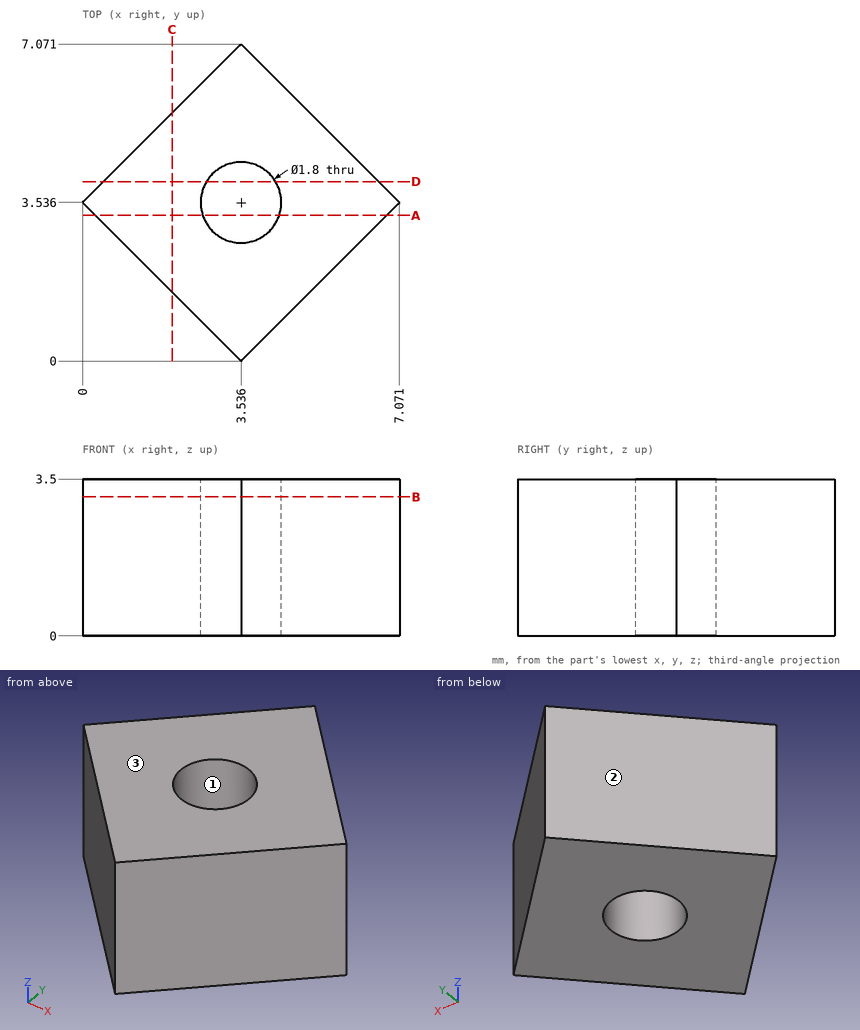
Here's the drawing with two shaded views (mm, measured from the low corner). I have some questions. Round coordinates to 2 decimals unless told otherwise and drop trailing zeros. Write each loop counter-clockwise with the first axis right and the second up, starting at its lowest first coordinate (ties: lowest second). Pieces come first, ordered by that corner, then holes. Notation, with made-up numbers: M 18,-10 L 22,-10 A29 cw 22,11 Z; hole C -12.5,-34.75 d2. An arc over 180 degrees is marked long. Use CSV: the item, a comma, the result in double quotes.
(1) I need wall thicknesses on line 1 along Y through (x, z) = (3.75, 3.3) (1 decimal); line 2 along Y through (x, z) = (3.25, 3.1) (1 decimal); line 3 along Y through (x, z) = (2.5, 0.85) (1 decimal). Which ranges of each line are inside material? Lowest first, please.
Check values:
line 1,"0.2 to 2.7, 4.4 to 6.9"
line 2,"0.3 to 2.7, 4.4 to 6.8"
line 3,"1 to 6"
(2) Imagine slicing it at B-B (z = 3.1). Write out the boundary of the cut face in (x, y) (1 decimal).
Check values:
outline,"M 0,3.5 L 3.5,0 L 7.1,3.5 L 3.5,7.1 Z; hole C 3.5,3.5 d1.8"
(3) Imagine slicing it at C-C (x = 2). Write out the boundary of the cut face in (y, z) (1 decimal).
Check values:
outline,"M 1.5,0 L 5.5,0 L 5.5,3.5 L 1.5,3.5 Z"
(4) I'm going to push flat-ended pins straight in: pin 1 (1.5 mm diameter, centred on x = 4, z = 1.5, fed in from +Y); pin 2 (1.6 mm diameter, centred on x = 3.54, y = 3.54, fed in from -Z); pin 3 (2 mm diameter, centred on y = 6, z = 3, fed in from +X) (1 decimal); pin 4 (2 mm diameter, centred on y = 5.5, z = 0.5, fed in from +X) (1 decimal). Where does each tip first touch, or does it pass through?
Check values:
pin 1,"y = 7.07"
pin 2,"through"
pin 3,"x = 5.6"
pin 4,"x = 6.1"
(5) Imagine slicing it at D-D (y = 4). Write out the boundary of the cut face in (x, z) (1 decimal), plus the area to 3 significant figures.
Check values:
outline,"M 0.5,0 L 2.8,0 L 2.8,3.5 L 0.5,3.5 Z; M 4.3,0 L 6.6,0 L 6.6,3.5 L 4.3,3.5 Z"
area,"16.1 mm^2"
(6) We'd pull the mould along X, two halves only. Please class the marked faces 1, 2 and 3: +X half, -X half, draft (parallel to the pull), parting line (faces both ways), or undercut.
Check values:
face 1,"undercut"
face 2,"-X half"
face 3,"draft"
(7) Imagine slicing it at A-A (y = 3.25). Write out the boundary of the cut face in (x, z) (1 decimal).
Check values:
outline,"M 0.3,0 L 2.7,0 L 2.7,3.5 L 0.3,3.5 Z; M 4.4,0 L 6.8,0 L 6.8,3.5 L 4.4,3.5 Z"
